Design review of the part built by this model. Coordinates are the model's own, in mm. Give positions to 0.01 mm unless a question says otherwise; leave off trailing zeros. Write each loop counter-clockwise with the first axis right and the second up, starting at its lowest first coordinate (ties: lowest second). Pieces come first, ordered by that corner, then holes. Notation, with made-up numbers: M 31.5,-15 L 87.5,-15 A8 ccw 87.5,-8 Z; hole C 75,79.25 d4. An arc over 180 degrees is marked long. Answer in a Markdown table with one row per item.
```python
from build123d import *

# Parameters (mm, degrees)
F0_R          = 12.5
F1_DEPTH      = 860
F2_R          = 5
F3_DEPTH      = 12.501
F3_DEPTH_BACK = 12.501


with BuildPart() as f1:
    # F0 (on Right) → F1 (new body)
    with BuildSketch(Plane.YZ):
        Circle(F0_R)
    extrude(amount=F1_DEPTH)

    # F2 (on Top) → F3 (cut, two sides)
    with BuildSketch(Plane.XY) as f3_sk:
        with Locations((20, 0)):
            Circle(F2_R)
        with Locations((840, 0)):
            Circle(F2_R)
    extrude(amount=F3_DEPTH, mode=Mode.SUBTRACT)
    extrude(f3_sk.sketch, amount=-F3_DEPTH_BACK, mode=Mode.SUBTRACT)


solid = f1.part
```
1) Add section A-A (y = 0). Write out the cut boundary in (x, z).
Geometry says:
| item | result |
|---|---|
| outline | M 0,-12.5 L 15,-12.5 L 15,12.5 L 0,12.5 Z; M 25,-12.5 L 835,-12.5 L 835,12.5 L 25,12.5 Z; M 845,-12.5 L 860,-12.5 L 860,12.5 L 845,12.5 Z |
2) To check wall thickness, follow probe 1 along X at (y, z) = (0, 3.25); probe 2 along Y at (x, z) = (20, 4.25); probe 3 along Z at (x, y) = (518, 0.5). State the ranges of each line that lie inside material, in increasing order. Write a range as [from, to].
Geometry says:
| item | result |
|---|---|
| probe 1 | [0, 15], [25, 835], [845, 860] |
| probe 2 | [-11.76, -5], [5, 11.76] |
| probe 3 | [-12.49, 12.49] |
3) Add section B-B (z = 8). Write out the cut boundary in (x, y).
Geometry says:
| item | result |
|---|---|
| outline | M 0,-9.6 L 860,-9.6 L 860,9.6 L 0,9.6 Z; hole C 20,0 d10; hole C 840,0 d10 |
4) Insertion check: P1, Ø8, axis at x = 840, y = 0, coming from the -Z side (3 decimals); P2, Ø3, axis at x = 481, z = -5.5, coming from the +Y side; P3, Ø12, axis at x = 613.5, y = 6.5, coming from the +Z side; P4, Ø3, axis at x = 312.5, z = 9, coming from the +Y side. Each pin has a flat end and moves straight along its axis. Give the tip position at first contact, or say it passes through.
Geometry says:
| item | result |
|---|---|
| P1 | through |
| P2 | y = 11.84 |
| P3 | z = 12.49 |
| P4 | y = 10 |
5) Add section C-C (x = 499.5). Write out the cut boundary in (y, z), and give its area (3 significant figures).
Geometry says:
| item | result |
|---|---|
| outline | C 0,0 d25 |
| area | 491 mm^2 |
